Study the drawing (mm; zero at the part's minimum x, y, z) and answer. A direction names the side the tool comes from. Round coordinates to 2 decimals unless told otherwise and drop trailing zeros. Write each loop counter-clockwise with the first axis right and the second up, starting at its lowest first coordinate (ties: lowest second). Pieces come first, ordered by that corner, then holes. Notation, with made-up numbers: (2.25, 24.25) - (50.25, 24.25) arc R34 ccw to (50.25, 56.25) - close; hole circle Ø9 at (-4, 88.25). An arc over 180 degrees is marked (long way). Return JSON: item names as keys, results as strings. Group by question number.
(1) Which of the six approach directions +Z, -Z, +X, -X, +Y, -Y give full straight-line access (tool end or side, diameter ignored) to the marked faces 1 and 2?
(2) Section B-B, the plane x = 80 is taken. Write down the section's boundary in (y, z).
(3) Section A-A, the plane y = 88 is taken. Write down the section's boundary in (x, z), then the cut area to 3 significant figures.
(4) This flat-tipped pin is pushed along its axis until it touches: pin 1 (12.5 mm diameter, centred on x = 90, y = 37.5, fed in from +Z). Where does it stop, or does it pass through?
(5) Find the intervals of material crossed by line 1 along Y through (x, z) = (80, 15.5); line 2 along Y through (x, z) = (80, 9.25); line 3 along Z through (x, y) = (106.5, 100.5), in increasing order. Write a range as [from, to].
(6) Section C-C, the plane x = 118 is taken. Write down the section's boundary in (y, z), then the cut area to 3 significant figures.
(7) Determine the mould class of the marked faces 3 and 4 for opening direction X: +X half, -X half, draft (parallel to the pull), parting line (faces both ways), or undercut.
(8) Section D-D, the plane z = 4 is taken. Write down the section's boundary in (x, y).
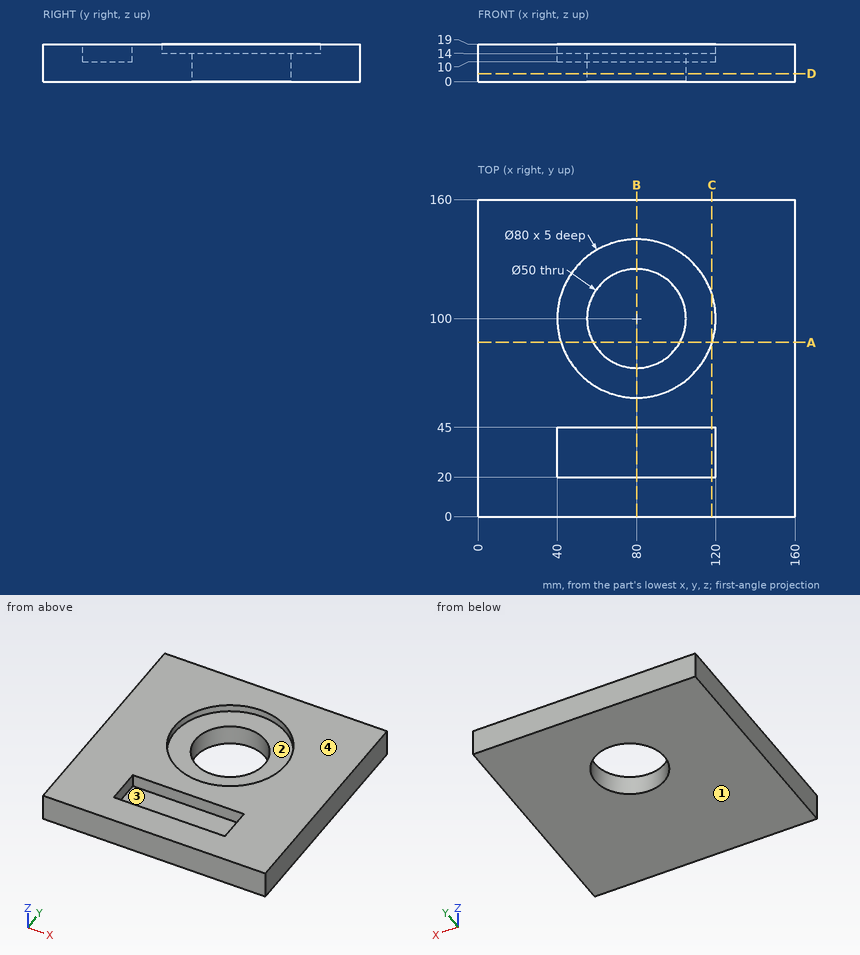
Working result:
{
 "1": {"face 1": "-Z, +X, -X, +Y, -Y", "face 2": "+Z"},
 "2": {"outline": "(0, 0) - (75, 0) - (75, 14) - (60, 14) - (60, 19) - (45, 19) - (45, 10) - (20, 10) - (20, 19) - (0, 19) - close; (125, 0) - (160, 0) - (160, 19) - (140, 19) - (140, 14) - (125, 14) - close"},
 "3": {"outline": "(0, 0) - (58.07, 0) - (58.07, 14) - (41.84, 14) - (41.84, 19) - (0, 19) - close; (101.93, 0) - (160, 0) - (160, 19) - (118.16, 19) - (118.16, 14) - (101.93, 14) - close", "area": "2,040 mm^2"},
 "4": {"pin 1": "stops at z = 10"},
 "5": {"line 1": "y = [0, 20], [45, 60], [140, 160]", "line 2": "y = [0, 75], [125, 160]", "line 3": "z = [0, 14]"},
 "6": {"outline": "(0, 0) - (160, 0) - (160, 19) - (112.49, 19) - (112.49, 14) - (87.51, 14) - (87.51, 19) - (45, 19) - (45, 10) - (20, 10) - (20, 19) - (0, 19) - close", "area": "2,690 mm^2"},
 "7": {"face 3": "undercut", "face 4": "draft"},
 "8": {"outline": "(0, 0) - (160, 0) - (160, 160) - (0, 160) - close; hole circle Ø50 at (80, 100)"}
}
